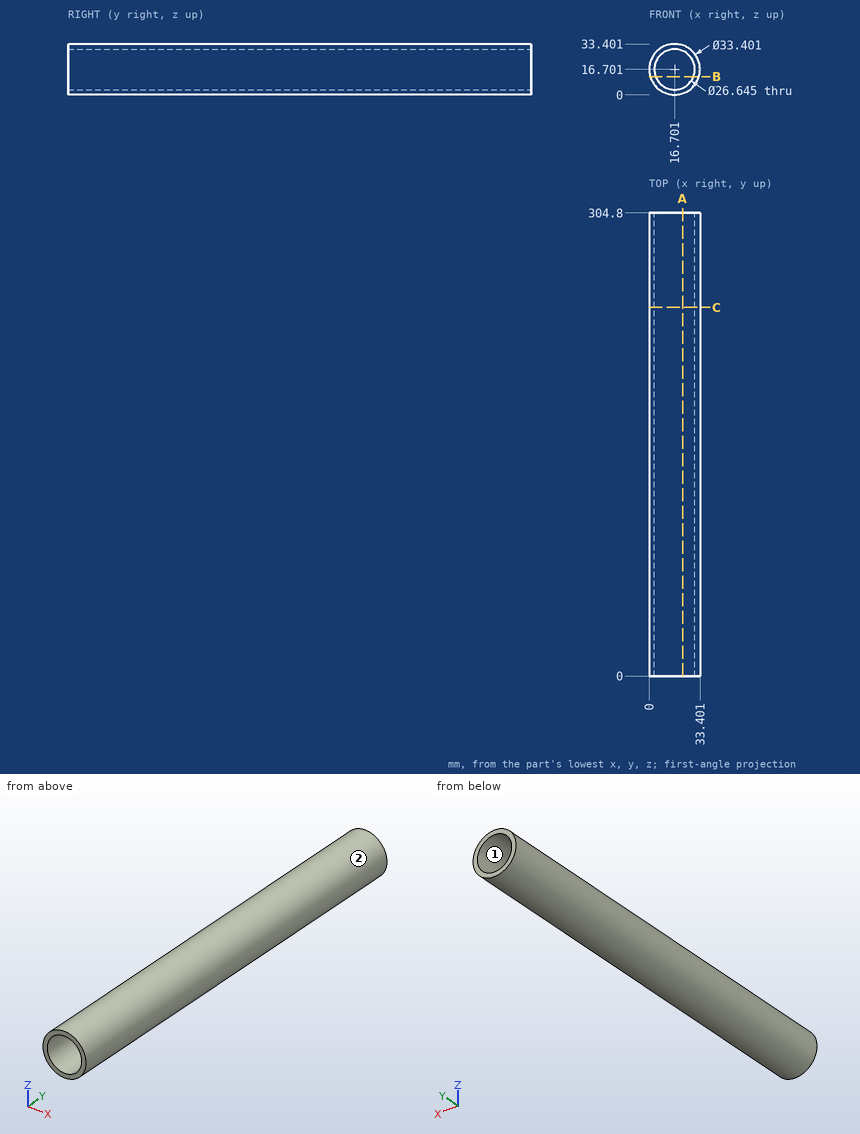
Can you work these out from the drawing? Everything is in mm from the part's minimum corner. Coordinates: 2 decimals unless noted, no trailing zeros. Order: outer loops, then holes, each group sorted by start corner. A loop starts at its lowest first (then second) coordinate and runs counter-clockwise, first axis right, second up. Notation, with made-up numbers: (9.5, 20) -> (25.5, 20) arc R10 cw to (25.5, 28) -> close; hole circle Ø7 at (-37, 14). An arc over 180 degrees is marked (long way). Return JSON: item names as keys, results as strings.
1) If we section it at B-B on z = 12: List the corners of the cut face in (x, y) for me (1 decimal), plus the area to 3 significant figures.
Conclusion:
{"outline": "(0.7, 0) -> (4.2, 0) -> (4.2, 304.8) -> (0.7, 304.8) -> close; (29.2, 0) -> (32.7, 0) -> (32.7, 304.8) -> (29.2, 304.8) -> close", "area": "2,170 mm²"}
2) If we section it at A-A on x = 22: List the corners of the cut face in (y, z) for me.
Conclusion:
{"outline": "(0, 0.86) -> (304.8, 0.86) -> (304.8, 4.48) -> (0, 4.48) -> close; (0, 28.92) -> (304.8, 28.92) -> (304.8, 32.54) -> (0, 32.54) -> close"}
3) Thinking about a two-plate mould opening in X: for the marked faces 1 and 2, which applies, +X half, -X half, draft (parallel to the pull), parting line (faces both ways), or undercut?
Conclusion:
{"face 1": "undercut", "face 2": "parting line"}
4) If we section it at C-C on y = 242.5: List the corners of the cut face in (x, z) for me (1 decimal).
Conclusion:
{"outline": "circle Ø33.4 at (16.7, 16.7); hole circle Ø26.6 at (16.7, 16.7)"}
5) If I drill on probe 1 along X at (y, z) = (284, 17.5); probe 2 along Z at (x, y) = (14, 57) (1 decimal); probe 3 along X at (y, z) = (281, 23) (1 decimal), over which ranges is the centre line in solid material (lowest first)?
Conclusion:
{"probe 1": "x = 0.02 to 3.4, 30 to 33.38", "probe 2": "z = 0.2 to 3.7, 29.7 to 33.2", "probe 3": "x = 1.2 to 5, 28.4 to 32.2"}
6) I'm going to push flat-ended pins straight in: P1, Ø6, axis at x = 21, y = 264, coming from the -Z side; P2, Ø2, axis at y = 138, z = 19, coming from the +X side; P3, Ø8, axis at x = 7, y = 180, coming from the +Z side. Where does each tip first touch, or does it pass through?
Conclusion:
{"P1": "stops at z = 0.05", "P2": "stops at x = 33.35", "P3": "stops at z = 32.4"}
